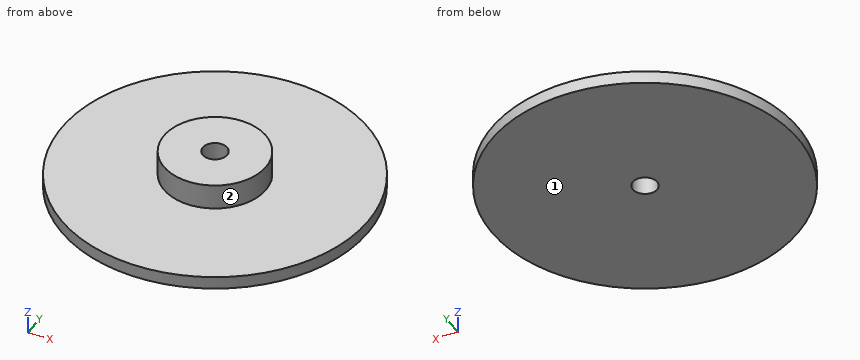
```python
from build123d import *

# Parameters (mm, degrees)
F0_R     = 19.05
F1_DEPTH = 1.5875
F2_R     = 6.35
F3_DEPTH = 3.175
F4_R     = 1.524
F5_DEPTH = 4.7635


with BuildPart() as f1:
    # F0 (on Top) → F1 (new body)
    with BuildSketch(Plane.XY):
        Circle(F0_R)
    extrude(amount=F1_DEPTH)

    # F2 (on face) → F3 (join)
    with BuildSketch(Plane.XY.offset(1.5875)):
        Circle(F2_R)
    extrude(amount=F3_DEPTH)

    # F4 (on face) → F5 (cut, through all)
    with BuildSketch(Plane.XY.offset(4.7625)):
        Circle(F4_R)
    extrude(amount=-F5_DEPTH, mode=Mode.SUBTRACT)


solid = f1.part
```
Geometry: final body of the model. Coordinates: model frame, mm. Face numbers are marked on the shaded views. A direction names the side the tool comes from. Round coordinates to 2 decimals unless told otherwise and drop trailing zeros. Write each loop counter-clockwise with the first axis right and the second up, starting at its lowest first coordinate (ties: lowest second). Pieces come first, ordered by that corner, then holes. Notation, with made-up numbers: (86, 79.5) -> (138, 79.5) arc R11 cw to (138, 87.5) -> close; hole circle Ø8 at (40.5, 55). An arc over 180 degrees is marked (long way). Use CSV: the item, a comma, the result in double quotes. Start each with the question number.
Q1. Line query: L1, parallel to Y at x = 0, z = 1.25; L2, parallel to Y at x = 0, z = 3.5; L3, parallel to Z at x = -5, y = -8. Output: solid intervals per line, ascending.
Q2. Section D-D (y = 12). Return loops of the section in (x, z).
Q3. Section C-C (x = -5). Return loops of the section in (y, z).
Q4. Section A-A (x = 0). Return loops of the section in (y, z), plus the area to 3 significant figures.
Q5. First-contact query: pin 1 Ø1.5 at (y, z) = (11.5, 2.5) entering from -X; pin 2 Ø1 at (x, z) = (-12, 2) entering from +Y; pin 3 Ø2 at (x, z) = (-2.5, 4) entering from -Y. Flat tips, straight axial feed; report the tip coordinate or a pass-through.
Q6. Reachability of the marked faces 1 and 2 from +Z, -Z, +X, -X, +Y, -Y: full face, straight path, thin tool, end or side. Return the list, or none.
Result sheet:
1,L1,"-19.05 to -1.52, 1.52 to 19.05"
1,L2,"-6.35 to -1.52, 1.52 to 6.35"
1,L3,"0 to 1.59"
2,outline,"(-14.8, 0) -> (14.8, 0) -> (14.8, 1.59) -> (-14.8, 1.59) -> close"
3,outline,"(-18.38, 0) -> (18.38, 0) -> (18.38, 1.59) -> (3.91, 1.59) -> (3.91, 4.76) -> (-3.91, 4.76) -> (-3.91, 1.59) -> (-18.38, 1.59) -> close"
4,outline,"(-19.05, 0) -> (-1.52, 0) -> (-1.52, 4.76) -> (-6.35, 4.76) -> (-6.35, 1.59) -> (-19.05, 1.59) -> close; (1.52, 0) -> (19.05, 0) -> (19.05, 1.59) -> (6.35, 1.59) -> (6.35, 4.76) -> (1.52, 4.76) -> close"
4,area,"86.3 mm²"
5,pin 1,"through"
5,pin 2,"y = 15.02"
5,pin 3,"y = -6.17"
6,face 1,"-Z, +X, -X, +Y, -Y"
6,face 2,"+Z"
